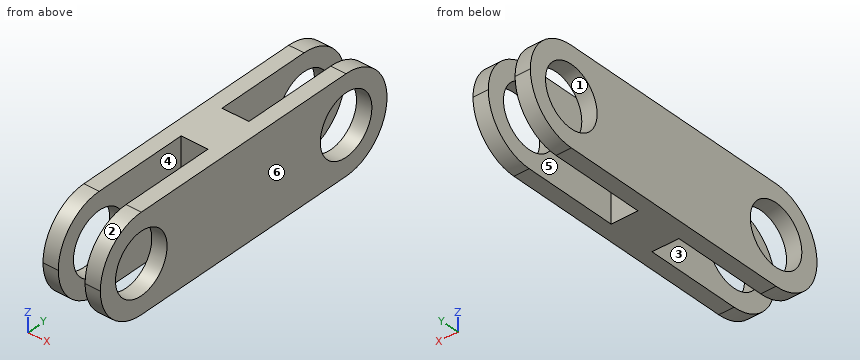
```python
from build123d import *

# Parameters (mm, degrees)
F1_DEPTH   = 0.889
F3_DEPTH   = 6.35
F4_R       = 3.17499
F7_D       = 4
F7_ON_F6_D = 4


# Not quite as in the source:
# - a fillet or chamfer is up to 0.001 mm smaller than in the source, because OpenCascade refuses the exact size
# - a feature names something its author has since deleted; it is built from what else it names


with BuildPart() as f1:
    # F0 (on Right) → F1 (new body, symmetric)
    with BuildSketch(Plane.YZ):
        Polygon((1.5875, 3.175), (-1.5875, 3.175), (-1.5875, 0), (0, 0), (1.5875, 0), align=None)
        Polygon((0, 0), (-1.5875, 0), (-1.5875, -3.175), (1.5875, -3.175), (1.5875, 0), align=None)
    extrude(amount=F1_DEPTH, both=True)

    # F2 (on face) → F3 (join)
    with BuildSketch(Plane(origin=(0, 0, -3.175), x_dir=(1, 0, 0), z_dir=(0, 0, -1))):
        Polygon((0.889, 0), (1.905, 0), (1.905, 11.1125), (0.889, 11.1125), (0.889, 1.5875), (-0.889, 1.5875), (-0.889, 11.1125), (-1.905, 11.1125), (-1.905, 0), (-0.889, 0), (0, 0), align=None)
        Polygon((1.905, -11.1125), (1.905, 0), (0.889, 0), (0, 0), (-0.889, 0), (-1.905, 0), (-1.905, -11.1125), (-0.889, -11.1125), (-0.889, -1.5875), (0.889, -1.5875), (0.889, -11.1125), align=None)
    extrude(amount=-F3_DEPTH)

    # F4 (radius 3.175 in the source; OpenCascade refuses exactly that, so slightly less here)
    f4_edges = [f1.edges().sort_by_distance(p)[0] for p in [
        (1.397, -11.1125, 3.175),
        (-1.397, -11.1125, 3.175),
        (1.397, -11.1125, -3.175),
        (-1.397, -11.1125, -3.175),
        (-1.397, 11.1125, -3.175),
        (1.397, 11.1125, -3.175),
        (1.397, 11.1125, 3.175),
        (-1.397, 11.1125, 3.175),
    ]]
    fillet(f4_edges, radius=F4_R)

    # F7 (through all)
    with Locations(Plane.YZ.offset(1.905)):
        with Locations((-7.9375, 0)):
            Hole(F7_D / 2)

    # F7 on F6 (through all)
    with Locations(Plane.YZ.offset(1.905)):
        with Locations((7.9375, 0)):
            Hole(F7_ON_F6_D / 2)


solid = f1.part
```
Here's how the part is built. I have some questions about the finished solid (model axes, mm). Face numbers are marked on the shaded views. A direction names the side the tool comes from. Give positions to 0.01 mm unless a question says otherwise; leave off trailing zeros. Order: outer loops, then holes, each group sorted by start corner. A loop starts at its lowest first (then second) coordinate and runs counter-clockwise, first axis right, second up. Notation, with made-up numbers: (81.5, 2.25) - (133.5, 2.25) arc R25 ccw to (133.5, 17.25) - close; hole circle Ø1 at (-18.5, -3). An arc over 180 degrees is marked (long way). Answer as a JSON object with one key per item and string values. Group by question number.
Item 1: If we section it at B-B on y = -3: Please give me the cut outline in (x, z) (3 decimals).
Item 2: Which directions (+Z, -Z, +X, -X, +Y, -Y) give clear straight access to the entire face, cutting with the end or side of a thin tool? Please do the marked faces 4, 5 and 6.
Item 3: For P1, Ø3.5, axis at y = -7.94, z = 0, coming from the -X side; P2, Ø0.9, axis at x = 0, z = -1, coming from the -Y side; P3, Ø2, axis at x = 1.5, z = 2, coming from the -Y side; P4, Ø0.9, axis at x = 0, z = 0.5, coming from the +Y side, each with a flat end and sliding along its axis, tell me the tip position at first contact or that it passes through.
Item 4: If we section it at A-A on x = -1.1: Give the number of separate pieces and of enclosed holes in the cut face, and give its area (3 significant figures).
Item 5: If we section it at C-C on x = 0.5: Please give me the cut outline in (y, z) (1 decimal), and give its area (3 significant figures).
Item 6: Please list where these lines run through material, in increasing order: probe 1 along X at (y, z) = (-5, 1.25) (3 decimals); probe 2 along Y at (x, z) = (0, -2.5); probe 3 along Z at (x, y) = (-1.35, 8).
Item 7: If we mould it in two halves opening along Y, with no side actions, what happens to the marked faces 1, 2 and 3? For each: pulls with the +Y half, pulls with the -Y half, needs draft (parallel to the pull), parting line crosses it, or undercut.
Result set:
{
 "1": {"outline": "(-1.905, -3.175) - (-0.889, -3.175) - (-0.889, 3.175) - (-1.905, 3.175) - close; (0.889, -3.175) - (1.905, -3.175) - (1.905, 3.175) - (0.889, 3.175) - close"},
 "2": {"face 4": "+Z, -Z, -Y", "face 5": "+Z, -Z, +Y", "face 6": "+Z, -Z, +X, +Y, -Y"},
 "3": {"P1": "through", "P2": "y = -1.59", "P3": "y = -10.95", "P4": "y = 1.59"},
 "4": {"separate pieces": "1", "enclosed holes": "2", "area": "107 mm²"},
 "5": {"outline": "(-1.6, -3.2) - (1.6, -3.2) - (1.6, 3.2) - (-1.6, 3.2) - close", "area": "20.2 mm²"},
 "6": {"probe 1": "-1.905 to -0.889, 0.889 to 1.905", "probe 2": "-1.59 to 1.59", "probe 3": "-3.17 to -2, 2 to 3.17"},
 "7": {"face 1": "undercut", "face 2": "pulls with the -Y half", "face 3": "needs draft"}
}
